```python
from build123d import *

# Parameters (mm, degrees)
SKETCH1_W           = 42.5
SKETCH1_H           = 42.5
BOSS_EXTRUDE1_DEPTH = 8
SKETCH2_R           = 1.7
SKETCH2_R_2         = 11.5
CUT_EXTRUDE1_DEPTH  = 35
BOSS_EXTRUDE2_DEPTH = 22
BOSS_EXTRUDE3_REACH = 52.416
SKETCH5_W           = 10
SKETCH5_H           = 42.5
FILLET1_R           = 4
FILLET2_R           = 4
CHAMFER2_SIZE       = 5
CUT_EXTRUDE2_DEPTH  = 2.6
SKETCH7_R           = 1.7
CUT_EXTRUDE3_DEPTH  = 10.6
CHAMFER3_SIZE       = 5
FILLET3_R           = 1
FILLET4_R           = 1
FILLET5_R           = 0.5


# Some blends are built 0.0001 mm under size
with BuildPart() as part:
    # Sketch1 → Boss-Extrude1 (new body)
    with BuildSketch(Plane(origin=(0, 0, 0), x_dir=(0, 0, -1), z_dir=(1, 0, 0))):
        Rectangle(SKETCH1_W, SKETCH1_H)
    extrude(amount=BOSS_EXTRUDE1_DEPTH)

    # Sketch2 → Cut-Extrude1 (cut)
    with BuildSketch(Plane(origin=(8, 0, 0), x_dir=(0, 0, -1), z_dir=(1, 0, 0))):
        with Locations((-15.5, 15.5)):
            Circle(SKETCH2_R)
        with Locations((15.5, 15.5)):
            Circle(SKETCH2_R)
        with Locations((-15.5, -15.5)):
            Circle(SKETCH2_R)
        with Locations((15.5, -15.5)):
            Circle(SKETCH2_R)
        Circle(SKETCH2_R_2)
    extrude(amount=-CUT_EXTRUDE1_DEPTH, mode=Mode.SUBTRACT)

    # Sketch3 → Boss-Extrude2 (add)
    with BuildSketch(Plane(origin=(8, 0, 0), x_dir=(0, 0, -1), z_dir=(1, 0, 0))):
        with BuildLine():
            Line((-19.5, -13.25), (-21.25, -13.25))
            Line((-21.25, -13.25), (-21.25, -21.25))
            Line((-21.25, -21.25), (21.25, -21.25))
            Line((21.25, -21.25), (21.25, -13.25))
            Line((21.25, -13.25), (19.5, -13.25))
            Line((19.5, -13.25), (19.5, -15.5))
            ThreePointArc((19.5, -15.5), (15.5, -19.5), (11.5, -15.5))
            Line((11.5, -15.5), (11.5, -13.25))
            Line((11.5, -13.25), (-11.5, -13.25))
            Line((-11.5, -13.25), (-11.5, -15.5))
            ThreePointArc((-11.5, -15.5), (-15.5, -19.5), (-19.5, -15.5))
            Line((-19.5, -15.5), (-19.5, -13.25))
        make_face()
    extrude(amount=BOSS_EXTRUDE2_DEPTH)

    # Boss-Extrude3: up to this face of the body (flat: up to its plane)
    boss_extrude3_end = Plane(part.part.faces().sort_by_distance((15, -21.25, 0))[0])
    # Sketch5 → Boss-Extrude3 (add, up to the picked face)
    with BuildSketch(Plane(origin=(0, -13.25, 0), x_dir=(1, 0, 0), z_dir=(0, 1, 0)), mode=Mode.PRIVATE) as boss_extrude3_sk1:
        with Locations((25, 0)):
            Rectangle(SKETCH5_W, SKETCH5_H)
    boss_extrude3_tool1 = split(extrude(boss_extrude3_sk1.sketch, amount=-BOSS_EXTRUDE3_REACH, mode=Mode.PRIVATE), bisect_by=boss_extrude3_end, keep=Keep.BOTH, mode=Mode.PRIVATE)
    add(boss_extrude3_tool1.solids().sort_by(Axis((25, -13.25, 0), (0, -1, 0)))[0])

    # Fillet1
    fillet1_edges = [part.edges().sort_by_distance(p)[0] for p in [
        (20, -14.375, 11.5),
        (20, -19.5, 15.5),
        (20, -14.375, 19.5),
    ]]
    fillet(fillet1_edges, radius=FILLET1_R - 0.0001)  # a hair under: the kernel refuses the full size

    # Fillet2
    fillet2_edges = [part.edges().sort_by_distance(p)[0] for p in [
        (20, -14.375, -11.5),
        (20, -19.5, -15.5),
        (20, -14.375, -19.5),
    ]]
    fillet(fillet2_edges, radius=FILLET2_R - 0.0001)  # a hair under: the kernel refuses the full size

    # Chamfer2
    # the kernel refuses this chamfer: 5 mm, written as the material it adds along each edge
    with BuildSketch(Plane(origin=(8, -13.25, -21.25), x_dir=(0.9996219169112968, -0.027495876610586317, 0), z_dir=(0, 0, 1)), Plane(origin=(8, -13.25, 19.5), x_dir=(0.9996219169112968, -0.027495876610586317, 0), z_dir=(0, 0, 1))) as chamfer2_piece_1:
        Polygon((CHAMFER2_SIZE * 0.999621916911, CHAMFER2_SIZE * 0.0274958766106), (-CHAMFER2_SIZE * 0.0274958766106, CHAMFER2_SIZE * 0.999621916911), (0, 0), align=None)
    extrude(amount=1.75)
    with BuildSketch(Plane(origin=(8, -13.25, -21.25), x_dir=(0.9996219169112968, -0.027495876610586317, 0), z_dir=(0, 0, 1))) as chamfer2_piece_2_section:
        Polygon((CHAMFER2_SIZE * 0.999621916911, CHAMFER2_SIZE * 0.0274958766106), (-CHAMFER2_SIZE * 0.0274958766106, CHAMFER2_SIZE * 0.999621916911), (0, 0), align=None)
    chamfer2_piece_2 = extrude(amount=14.60841494, mode=Mode.PRIVATE)
    chamfer2_piece_2 = split(chamfer2_piece_2, bisect_by=Plane(origin=(9.660792582, -11.623563686, -11.5), z_dir=(0, 0, 1)), keep=Keep.TOP, mode=Mode.PRIVATE)
    chamfer2_piece_2 = chamfer2_piece_2 - Plane(origin=(9.660792582, 0, 0), x_dir=(0, 0, -1), z_dir=(1, 0, 0)) * Cylinder(11.5, 50, mode=Mode.PRIVATE)
    add(chamfer2_piece_2)
    with BuildSketch(Plane(origin=(8, -13.25, 6.64158506), x_dir=(0.9996219169112968, -0.027495876610586313, 0), z_dir=(0, 0, 1))) as chamfer2_piece_3_section:
        Polygon((CHAMFER2_SIZE * 0.999621916911, CHAMFER2_SIZE * 0.0274958766106), (-CHAMFER2_SIZE * 0.0274958766106, CHAMFER2_SIZE * 0.999621916911), (0, 0), align=None)
    chamfer2_piece_3 = extrude(amount=14.60841494, mode=Mode.PRIVATE)
    chamfer2_piece_3 = split(chamfer2_piece_3, bisect_by=Plane(origin=(9.660792582, -11.623563686, 11.5), z_dir=(0, 0, -1)), keep=Keep.TOP, mode=Mode.PRIVATE)
    chamfer2_piece_3 = chamfer2_piece_3 - Plane(origin=(9.660792582, 0, 0), x_dir=(0, 0, -1), z_dir=(1, 0, 0)) * Cylinder(11.5, 50, mode=Mode.PRIVATE)
    add(chamfer2_piece_3)
    with BuildSketch(Plane(origin=(8, -13.25, -24.35841494), x_dir=(0.9996219169112968, -0.027495876610586313, 0), z_dir=(0, 0, 1))) as chamfer2_piece_4_section:
        Polygon((CHAMFER2_SIZE * 0.999621916911, CHAMFER2_SIZE * 0.0274958766106), (-CHAMFER2_SIZE * 0.0274958766106, CHAMFER2_SIZE * 0.999621916911), (0, 0), align=None)
    chamfer2_piece_4 = extrude(amount=35.85841494, mode=Mode.PRIVATE)
    chamfer2_piece_4 = split(chamfer2_piece_4, bisect_by=Plane(origin=(9.648968134, -11.601031866, -19.5), z_dir=(0, 0, -1)), keep=Keep.TOP, mode=Mode.PRIVATE)
    chamfer2_piece_4 = split(chamfer2_piece_4, bisect_by=Plane(origin=(9.648968134, -11.601031866, -21.25), z_dir=(0, 0, 1)), keep=Keep.TOP, mode=Mode.PRIVATE)
    add(chamfer2_piece_4)
    with BuildSketch(Plane(origin=(8, -13.25, -11.5), x_dir=(0.9996219169112968, -0.027495876610586317, 0), z_dir=(0, 0, 1))) as chamfer2_piece_5_section:
        Polygon((CHAMFER2_SIZE * 0.999621916911, CHAMFER2_SIZE * 0.0274958766106), (-CHAMFER2_SIZE * 0.0274958766106, CHAMFER2_SIZE * 0.999621916911), (0, 0), align=None)
    chamfer2_piece_5 = extrude(amount=23, mode=Mode.PRIVATE)
    chamfer2_piece_5 = chamfer2_piece_5 - Plane(origin=(9.815143963, 0, 0), x_dir=(0, 0, -1), z_dir=(1, 0, 0)) * Cylinder(11.5, 66, mode=Mode.PRIVATE)
    add(chamfer2_piece_5)
    with BuildSketch(Plane(origin=(8, -13.25, -11.5), x_dir=(0.9996219169112968, -0.027495876610586317, 0), z_dir=(0, 0, 1))) as chamfer2_piece_6_section:
        Polygon((CHAMFER2_SIZE * 0.999621916911, CHAMFER2_SIZE * 0.0274958766106), (-CHAMFER2_SIZE * 0.0274958766106, CHAMFER2_SIZE * 0.999621916911), (0, 0), align=None)
    chamfer2_piece_6 = extrude(amount=35.85841494, mode=Mode.PRIVATE)
    chamfer2_piece_6 = split(chamfer2_piece_6, bisect_by=Plane(origin=(9.648968134, -11.601031866, 19.5), z_dir=(0, 0, 1)), keep=Keep.TOP, mode=Mode.PRIVATE)
    chamfer2_piece_6 = split(chamfer2_piece_6, bisect_by=Plane(origin=(9.648968134, -11.601031866, 21.25), z_dir=(0, 0, -1)), keep=Keep.TOP, mode=Mode.PRIVATE)
    add(chamfer2_piece_6)

    # Sketch6 → Cut-Extrude2 (cut)
    with BuildSketch(Plane(origin=(0, -13.25, 0), x_dir=(1, 0, 0), z_dir=(0, 1, 0))):
        Polygon((25, 12.901368439), (27.9, 14.575684219), (27.9, 17.924315781), (25, 19.598631561), (22.1, 17.924315781), (22.1, 14.575684219), align=None)
        Polygon((25, -19.598631561), (27.9, -17.924315781), (27.9, -14.575684219), (25, -12.901368439), (22.1, -14.575684219), (22.1, -17.924315781), align=None)
    extrude(amount=-CUT_EXTRUDE2_DEPTH, mode=Mode.SUBTRACT)

    # Sketch7 → Cut-Extrude3 (cut)
    with BuildSketch(Plane(origin=(0, -15.85, 0), x_dir=(1, 0, 0), z_dir=(0, 1, 0))):
        with Locations(Location((25, 16.25, 0), (0, 0, 270))):
            Circle(SKETCH7_R)
        with Locations(Location((25, -16.25, 0), (0, 0, 270))):
            Circle(SKETCH7_R)
    extrude(amount=-CUT_EXTRUDE3_DEPTH, mode=Mode.SUBTRACT)

    # Chamfer3
    chamfer3_edges = [part.edges().sort_by_distance(p)[0] for p in [
        (4, 21.25, 21.25),
        (4, 21.25, -21.25),
    ]]
    chamfer(chamfer3_edges, length=CHAMFER3_SIZE)

    # Fillet3
    fillet3_edges = [part.edges().sort_by_distance(p)[0] for p in [
        (0, -2.5, 21.25),
        (30, -17.25, 21.25),
        (30, -17.25, -21.25),
        (0, -2.5, -21.25),
    ]]
    fillet(fillet3_edges, radius=FILLET3_R)

    # Fillet4
    fillet4_edges = [part.edges().sort_by_distance(p)[0] for p in [
        (8, 4, -21.25),
        (8, 4, 21.25),
    ]]
    fillet(fillet4_edges, radius=FILLET4_R)

    # Fillet5
    fillet5_edges = [part.edges().sort_by_distance(p)[0] for p in [
        (30, -21.25, 0),
        (15, -21.25, -21.25),
        (0, -21.25, 0),
        (15, -21.25, 21.25),
        (29.707106781, -21.25, 20.957106781),
        (0.292893219, -21.25, 20.957106781),
        (0.292893219, -21.25, -20.957106781),
        (29.707106781, -21.25, -20.957106781),
    ]]
    fillet(fillet5_edges, radius=FILLET5_R)


solid = part.part
```
CAD build for the part. Positions are in the model's coordinates, mm. A direction names the side the tool comes from. Round coordinates to 2 decimals unless told otherwise and drop trailing zeros. Write each loop counter-clockwise with the first axis right and the second up, starting at its lowest first coordinate (ties: lowest second). Pieces come first, ordered by that corner, then holes. Notation, with made-up numbers: (26.25, 53) - (74.25, 53) arc R13 ccw to (74.25, 78) - close; hole circle Ø7 at (33, 67.25). An arc over 180 degrees is marked (long way). Write item = value, one per line. Start each with the question number.
Q1. Band-saw the part on D-D (y = -10). Give the cut face in (x, z).
Q2. Drop flat-ended pins along their axis: pin 1 (3 mm diameter, centred on y = 15.5, z = 15.5, fed in from +X); pin 2 (2 mm diameter, centred on y = -15.5, z = 15.5, fed in from -X); pin 3 (6.5 mm diameter, centred on x = 25, z = -17, fed in from +Y); pin 4 (2 mm diameter, centred on y = -7.5, z = -10.5, fed in from +X). Give the stop position or say it passes through.
Q3. Which spindle directions (+Z, -Z, +X, -X, +Y, -Y) get a long thin tool onto all of the face, cutting with end or side? Do faces 4 (the flat face through (11, -13, 11.5)), 5 (the cylindrical face through (4.06, 14.85, -17.07)). Say none if no direction does.
Q4. Band-saw the part on C-C (y = 2). Give the cut face in (x, z), then the cut area to 3 significant figures.
Q5. Band-saw the part on A-A (y = 15.5). Give the cut face in (x, z), then the cut area to 3 significant figures.
Q6. Band-saw the part on B-B (z = -1). Give the cut face in (x, y).
Q7. Probe L1, parallel to Y at x = 5.5, z = -15.5; L2, parallel to Z at x = 25.25, y = -18; L3, parallel to Z at x = 5.75, y = 0. List the from-to ranges inside material, lowest first. Write a range as from..to.
Q8. Mould opens along Z. For faces 1 (the cylindrical face through (4.06, -16.15, 13.93)), 2 (the flat face through (11.65, -11.9, -0.16)), 3 (the flat face through (3.9, 18.8, -18.7)) say: pulls with the +Z half, pulls with the -Z half, needs draft (parallel to the pull), parting line crosses it, or undercut.
Answers below:
q1.outline = (0, -20.25) arc R1 ccw to (1, -21.25) - (9.75, -21.25) - (9.75, -19.5) - (8, -19.5) - (8, -11.5) - (9.75, -11.5) - (9.75, -5.68) - (0, -5.68) - close; (0, 5.68) - (9.75, 5.68) - (9.75, 11.5) - (8, 11.5) - (8, 19.5) - (9.75, 19.5) - (9.75, 21.25) - (1, 21.25) arc R1 ccw to (0, 20.25) - close
q2.pin_1 = through
q2.pin_2 = 19.87
q2.pin_3 = -13.25
q2.pin_4 = 8.25
q3.face_4 = +Y
q3.face_5 = +X, -X
q4.outline = (0, -20.25) arc R1 ccw to (1, -21.25) - (7, -21.25) arc R1 ccw to (8, -20.25) - (8, -11.32) - (0, -11.32) - close; (0, 11.32) - (8, 11.32) - (8, 20.25) arc R1 ccw to (7, 21.25) - (1, 21.25) arc R1 ccw to (0, 20.25) - close
q4.area = 158 mm2
q5.outline = (0, -20.25) arc R1 ccw to (1, -21.25) - (7, -21.25) arc R1 ccw to (8, -20.25) - (8, -17.2) - (0, -17.2) - close; (0, -13.8) - (8, -13.8) - (8, 13.8) - (0, 13.8) - close; (0, 17.2) - (8, 17.2) - (8, 20.25) arc R1 ccw to (7, 21.25) - (1, 21.25) arc R1 ccw to (0, 20.25) - close
q5.area = 285 mm2
q6.outline = (0, -20.75) arc R0.5 ccw to (0.5, -21.25) - (29.5, -21.25) arc R0.5 ccw to (30, -20.75) - (30, -13.25) - (13, -13.25) - (11.21, -11.46) - (0, -11.46) - close; (0, 11.46) - (8, 11.46) - (8, 21.25) - (0, 21.25) - close
q7.L1 = -21.25..-17.2, -13.8..13.8, 17.2..21.25
q7.L2 = -21.25..-17.93, -14.57..14.57, 17.93..21.25
q7.L3 = -21.25..-11.5, 11.5..21.25
q8.face_1 = undercut
q8.face_2 = needs draft
q8.face_3 = pulls with the -Z half
